Can you work these out from the model? Positions are in its coordinate system, mm. Coordinates: 2 decimals unless noted, no trailing zeros. Order: outer loops, then holes, each group sorted by start corner. A loop starts at its lowest first (then second) coordinate and runs counter-clockwise, first axis right, second up. Notation, with made-up numbers: (39.25, 62.5) -> (53.25, 62.5) arc R29 cw to (53.25, 101.5) -> close; hole circle Ø8 at (23, 82.5). An arc over 180 degrees is marked (long way). Answer in a Markdown table with one row per item. Add a question column.
1. Imagine slicing it at C-C on z = -20.5. Write out the boundary of the cut face in (x, y) (3 decimals), plus the area to 3 significant figures.
2. We'd pull the mould along X, two halves only. Please class faces 1 (the face through (0, -2, -56.031)), 2 (the face through (0.636, -1.565, -41.636)), 3 (the face through (-3.171, -1.565, 2.233)): pulls with the +X half, pulls with the -X half, needs draft (parallel to the pull), parting line crosses it, or undercut.
3. Will this pin go through, and if not, where does the flat tip stop? pin 1 (1.9 mm diameter, centred on x = 22.92, z = -53.03, fed in from -Y).
4. If I drill on line 1 along Z through (x, y) = (-19.05, -1.55); line 2 along X through (y, z) = (-2.8, 29.5); line 3 along X through (y, z) = (-0.35, 29), over which ranges is the centre line in solid material (lowest first)? Write a range as [from, to].
5. Imagine slicing it at A-A on x = 0. State how many separate pieces and enclosed holes the cut face has, plus the area to 3 significant figures.
6. Imagine slicing it at B-B on x = -19.05. Write out the boundary of the cut face in (y, z) (3 decimals), plus the area to 3 significant figures.
from build123d import *

# Parameters (mm, degrees)
F0_W     = 60.6
F0_H     = 128.5
F1_DEPTH = 3.175
F3_D     = 3.2
F5_D     = 5.87
F6_D     = 6.65
F7_D     = 3
F8_D     = 3.5


with BuildPart() as f1:
    # F0 (on Front) → F1 (new body)
    with BuildSketch(Plane.XZ):
        with Locations((0, 8.218851)):
            Rectangle(F0_W, F0_H)
    extrude(amount=F1_DEPTH)

    # F3 (through all)
    with Locations(Plane.XZ.offset(3.175)):
        with Locations((-22.8, -53.031149), (22.92, -53.031149), (22.92, 69.468851), (-22.8, 69.468851)):
            Hole(F3_D / 2)

    # F5 (through all)
    with Locations(Plane.XZ.offset(3.175)):
        with Locations((-23.622, -38.771149), (-23.622, -22.261149), (-11.811, -22.261149), (-11.811, -38.771149), (0, -22.261149), (0, -38.771149), (11.811, -22.261149), (11.811, -38.771149), (23.622, -22.261149), (23.622, -38.771149)):
            Hole(F5_D / 2)

    # F6 (through all)
    with Locations(Plane.XZ.offset(3.175)):
        with Locations((-19.05, 48.858851), (0, 39.333851), (19.05, 48.858851), (-19.05, 29.808851), (0, 20.283851), (19.05, 29.808851), (-19.05, 10.758851), (0, 1.233851), (19.05, 10.758851)):
            Hole(F6_D / 2)

    # F7 (through all)
    with Locations(Plane.XZ.offset(3.175)):
        with Locations((0, 60.288851)):
            Hole(F7_D / 2)

    # F8 (through all)
    with Locations(Plane.XZ.offset(3.175)):
        with Locations((0, 52.668851)):
            Hole(F8_D / 2)


solid = f1.part
Answers follow:
| question | item | result |
|---|---|---|
| 1 | outline | (-30.3, -3.175) -> (-25.97, -3.175) -> (-25.97, 0) -> (-30.3, 0) -> close; (-21.274, -3.175) -> (-14.159, -3.175) -> (-14.159, 0) -> (-21.274, 0) -> close; (-9.463, -3.175) -> (-2.348, -3.175) -> (-2.348, 0) -> (-9.463, 0) -> close; (2.348, -3.175) -> (9.463, -3.175) -> (9.463, 0) -> (2.348, 0) -> close; (14.159, -3.175) -> (21.274, -3.175) -> (21.274, 0) -> (14.159, 0) -> close; (25.97, -3.175) -> (30.3, -3.175) -> (30.3, 0) -> (25.97, 0) -> close |
| 1 | area | 118 mm² |
| 2 | face 1 | needs draft |
| 2 | face 2 | undercut |
| 2 | face 3 | undercut |
| 3 | pin 1 | passes through |
| 4 | line 1 | z = [-56.03, 7.43], [14.08, 26.48], [33.13, 45.53], [52.18, 72.47] |
| 4 | line 2 | x = [-30.3, -22.36], [-15.74, 15.74], [22.36, 30.3] |
| 4 | line 3 | x = [-30.3, -22.28], [-15.82, 15.82], [22.28, 30.3] |
| 5 | separate pieces | 8 |
| 5 | enclosed holes | 0 |
| 5 | area | 287 mm² |
| 6 | outline | (-3.175, -56.031) -> (0, -56.031) -> (0, 7.434) -> (-3.175, 7.434) -> close; (-3.175, 14.084) -> (0, 14.084) -> (0, 26.484) -> (-3.175, 26.484) -> close; (-3.175, 33.134) -> (0, 33.134) -> (0, 45.534) -> (-3.175, 45.534) -> close; (-3.175, 52.184) -> (0, 52.184) -> (0, 72.469) -> (-3.175, 72.469) -> close |
| 6 | area | 345 mm² |
